Input: part model. Units: mm. Frame: model coordinates. Face numbers are marked on the shaded views. A direction names the side the tool comes from. Give positions to 0.01 mm unless a question says otherwise; leave off trailing zeros. Loops run counter-clockwise (first coordinate to the right, second up) from the corner with the lowest first, then second, coordinate; pieces in that order, holes last. Notation, with made-up numbers: (-5, -9.75) -> (32, -9.75) arc R30 cw to (32, 17.25) -> close; hole circle Ø6 at (60, 57.25). An arc over 180 degrees is marked (long way). Answer as a JSON object with one key per item and string values.
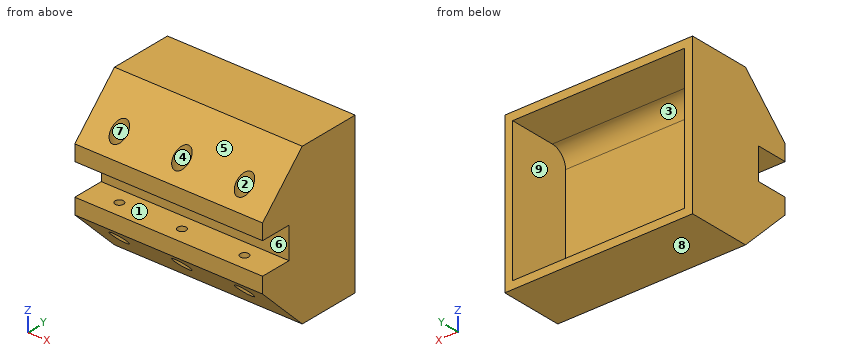
```python
from build123d import *

# Parameters (mm, degrees)
SKETCH1_W               = 152.4
SKETCH1_H               = 38.1
BOSS_EXTRUDE1_DEPTH     = 50.8
SKETCH2_W               = 25.4
SKETCH2_H               = 25.4
CUT_EXTRUDE1_DEPTH      = 152.4
BOSS_EXTRUDE2_DEPTH     = 152.4
CUT_EXTRUDE3_DEPTH      = 129.420802443
CUT_EXTRUDE3_DEPTH_BACK = 129.420802443
SKETCH6_R               = 6.35
SKETCH10_R              = 6.35
SKETCH10_R_2            = 3.429
BOSS_EXTRUDE3_DEPTH     = 10.16
CUT_EXTRUDE4_DEPTH      = 69.85


with BuildPart() as part:
    # Sketch1 → Boss-Extrude1 (new body)
    with BuildSketch(Plane.XY):
        Rectangle(SKETCH1_W, SKETCH1_H)
    extrude(amount=BOSS_EXTRUDE1_DEPTH)

    # Sketch2 → Cut-Extrude1 (cut)
    with BuildSketch(Plane.ZY.offset(76.2)):
        with Locations((25.4, -6.35)):
            Rectangle(SKETCH2_W, SKETCH2_H)
    extrude(amount=-CUT_EXTRUDE1_DEPTH, mode=Mode.SUBTRACT)

    # Sketch5 → Boss-Extrude2 (add)
    with BuildSketch(Plane(origin=(76.2, 0, 0), x_dir=(0, 0, -1), z_dir=(1, 0, 0))):
        Polygon((0, -19.05), (38.1, 19.05), (38.1, 69.85), (-88.9, 69.85), (-88.9, 19.05), (-50.8, -19.05), (-50.8, 19.05), (0, 19.05), align=None)
    extrude(amount=-BOSS_EXTRUDE2_DEPTH)

    # Sketch6 → Cut-Extrude3 (cut, two sides: drawn at the far end of the back side and taken through both)
    with BuildSketch(Plane(origin=(0, 0, 38.1), x_dir=(-1, 0, 0), z_dir=(0, 0, -1)).offset(-CUT_EXTRUDE3_DEPTH_BACK)):
        with Locations(Location((0, -6.35, 0), (0, 0, 90))):
            Circle(SKETCH6_R)
        with Locations(Location((-50.8, -6.35, 0), (0, 0, 90))):
            Circle(SKETCH6_R)
        with Locations(Location((50.8, -6.35, 0), (0, 0, 90))):
            Circle(SKETCH6_R)
    extrude(amount=CUT_EXTRUDE3_DEPTH + CUT_EXTRUDE3_DEPTH_BACK, mode=Mode.SUBTRACT)

    # Sketch10 → Boss-Extrude3 (add)
    # profile 1 of 3: a face of its own
    with BuildSketch(Plane.XY.offset(12.7)):
        with Locations(Location((-50.8, -6.35, 0), (0, 0, 90))):
            Circle(SKETCH10_R)
        with Locations((-50.8, -6.35)):
            Circle(SKETCH10_R_2, mode=Mode.SUBTRACT)
    # profile 2 of 3: a face of its own
    with BuildSketch(Plane.XY.offset(12.7)):
        with Locations(Location((0, -6.35, 0), (0, 0, 90))):
            Circle(SKETCH10_R)
        with Locations((0, -6.35)):
            Circle(SKETCH10_R_2, mode=Mode.SUBTRACT)
    # profile 3 of 3: a face of its own
    with BuildSketch(Plane.XY.offset(12.7)):
        with Locations(Location((50.8, -6.35, 0), (0, 0, 90))):
            Circle(SKETCH10_R)
        with Locations((50.8, -6.35)):
            Circle(SKETCH10_R_2, mode=Mode.SUBTRACT)
    boss_extrude3 = extrude(amount=-BOSS_EXTRUDE3_DEPTH)

    # Sketch11 → Cut-Extrude4 (cut, symmetric)
    with BuildSketch(Plane(origin=(0, 0, 0), x_dir=(0, 0, -1), z_dir=(1, 0, 0))):
        with BuildLine():
            Line((-82.55, 69.85), (-82.55, 31.75))
            ThreePointArc((-82.55, 31.75), (-78.830256121, 22.769743879), (-69.85, 19.05))
            Line((-69.85, 19.05), (19.05, 19.05))
            ThreePointArc((19.05, 19.05), (28.030256121, 22.769743879), (31.75, 31.75))
            Line((31.75, 31.75), (31.75, 69.85))
            Line((31.75, 69.85), (-82.55, 69.85))
        make_face()
    extrude(amount=CUT_EXTRUDE4_DEPTH, both=True, mode=Mode.SUBTRACT)

    # Mirror1: Boss-Extrude3 across plane
    add(boss_extrude3.mirror(Plane.XY.offset(25.4)))


solid = part.part
```
Q1. Ray query, line 1 along X through (y, z) = (-6.35, 57); line 2 along X through (y, z) = (27, 59.5); line 3 along Z through (x, y) = (-24, 44.5). Return the intervals inside material, ascending.
Evaluation:
{"line 1": "x = -76.2 to -57.15, -44.45 to -6.35, 6.35 to 44.45, 57.15 to 76.2", "line 2": "x = -76.2 to -69.85, 69.85 to 76.2", "line 3": "z = -38.1 to -31.75, 82.55 to 88.9"}
Q2. Section A-A, the plane y = 58. Return the cut outline in (x, z), then the cut area to 3 significant figures.
Evaluation:
{"outline": "(-76.2, -38.1) -> (76.2, -38.1) -> (76.2, 88.9) -> (-76.2, 88.9) -> close; hole (-69.85, -31.75) -> (69.85, -31.75) -> (69.85, 82.55) -> (-69.85, 82.55) -> close", "area": "3,390 mm2"}
Q3. Section B-B, the plane z = 46. Return the cut outline in (x, y).
Evaluation:
{"outline": "(-76.2, -19.05) -> (76.2, -19.05) -> (76.2, 69.85) -> (69.85, 69.85) -> (69.85, 19.05) -> (-69.85, 19.05) -> (-69.85, 69.85) -> (-76.2, 69.85) -> close; hole circle Ø6.86 at (-50.8, -6.35); hole circle Ø6.86 at (0, -6.35); hole circle Ø6.86 at (50.8, -6.35)"}
Q4. Section C-C, the plane x = 50.8. Give the number of separate pieces and of enclosed holes in the cut face, then the cut area to 3 significant figures.
Evaluation:
{"separate pieces": "3", "enclosed holes": "0", "area": "2,930 mm2"}
Q5. Pin query (flat end, axial travel): pin 1 (20.5 mm diameter, centred on x = -2, z = 23.5, fed in from -Y); pin 2 (11.5 mm diameter, centred on x = 50.8, y = -6.35, fed in from -Z); pin 3 (20.5 mm diameter, centred on x = -50.8, y = -6.35, fed in from -Z). Return the tip coordinate at first contact, or that it passes through.
Evaluation:
{"pin 1": "stops at y = 6.35", "pin 2": "stops at z = 2.54", "pin 3": "stops at z = -22.95"}
Q6. Draft query along Y for the marked faces 1, 2, 3 and 4. Return one class per face: +Y half, -Y half, draft (parallel to the pull), parting line (faces both ways), or undercut.
Evaluation:
{"face 1": "draft", "face 2": "undercut", "face 3": "+Y half", "face 4": "undercut"}
Q7. Access query for the marked faces 5, 6, 7, 8 and 9. Directions: +Z, -Z, +X, -X, +Y, -Y. A direction counts if a zero-diameter tool reaches every point of the face in a straight line with its end or side. Return the directions, or none.
Evaluation:
{"face 5": "+Z, +X, -X, -Y", "face 6": "+X, -X, -Y", "face 7": "+Z", "face 8": "-Z, +X, -X, +Y, -Y", "face 9": "+Y"}
